The model under review builds one solid part; all positions refer to its coordinate system, in mm. A direction names the side the tool comes from. Coordinates: 2 decimals unless noted, no trailing zeros. Order: outer loops, then holes, each group sorted by start corner. A loop starts at its lowest first (then second) coordinate and runs counter-clockwise, first axis right, second up. Notation, with made-up numbers: (59.25, -20.75) -> (86.25, -20.75) arc R18 ccw to (86.25, -4.75) -> close; hole circle Ø3 at (32, 89). An arc over 180 degrees is marked (long way). Put each result on its own line as item: value.
from build123d import *

# Parameters (mm, degrees)
JOTYY_MIRRORED_START         = -10
JOTYY_MIRRORED_OUTLINE_W     = 53.8
JOTYY_MIRRORED_OUTLINE_H     = 36
JOTYY_MIRRORED_OUTLINE_R     = 2.1
JOTYY_MIRRORED_OUTLINE_R_2   = 11
JOTYY_MIRRORED_DEPTH         = 10
JOTYY_MIRRORED_2_OUTLINE_R   = 11
JOTYY_MIRRORED_2_OUTLINE_R_2 = 4
JOTYY_MIRRORED_2_DEPTH       = 2.5
SKETCH1_R                    = 4
CUT_EXTRUDE1_DEPTH           = 10
CUT_EXTRUDE2_DEPTH           = 58.009529002


# Read off the part's stored shape, not the designer's step: jotyy_Mirrored
with BuildPart() as part:
    # jotyy_Mirrored outline → jotyy_Mirrored (new body)
    with BuildSketch(Plane.XY.offset(JOTYY_MIRRORED_START)):
        with Locations((-26.9, 20)):
            Rectangle(JOTYY_MIRRORED_OUTLINE_W, JOTYY_MIRRORED_OUTLINE_H)
        with Locations((-47.5, 7.5)):
            Circle(JOTYY_MIRRORED_OUTLINE_R, mode=Mode.SUBTRACT)
        with Locations((-22.5, 7.5)):
            Circle(JOTYY_MIRRORED_OUTLINE_R, mode=Mode.SUBTRACT)
        with Locations((-5, 7.5)):
            Circle(JOTYY_MIRRORED_OUTLINE_R, mode=Mode.SUBTRACT)
        with Locations((-35, 20)):
            Circle(JOTYY_MIRRORED_OUTLINE_R_2, mode=Mode.SUBTRACT)
        with Locations((-47.5, 32.5)):
            Circle(JOTYY_MIRRORED_OUTLINE_R, mode=Mode.SUBTRACT)
        with Locations((-22.5, 32.5)):
            Circle(JOTYY_MIRRORED_OUTLINE_R, mode=Mode.SUBTRACT)
        with Locations((-5, 32.5)):
            Circle(JOTYY_MIRRORED_OUTLINE_R, mode=Mode.SUBTRACT)
    extrude(amount=JOTYY_MIRRORED_DEPTH)

    # jotyy_Mirrored 2 outline → jotyy_Mirrored 2 (add)
    with BuildSketch(Plane.XY.offset(JOTYY_MIRRORED_START)):
        with Locations((-35, 20)):
            Circle(JOTYY_MIRRORED_2_OUTLINE_R)
        with Locations((-35, 20)):
            Circle(JOTYY_MIRRORED_2_OUTLINE_R_2, mode=Mode.SUBTRACT)
    extrude(amount=JOTYY_MIRRORED_2_DEPTH)

    # Sketch1 → Cut-Extrude1 (cut)
    with BuildSketch(Plane.XY):
        with Locations((-10, 20)):
            Circle(SKETCH1_R)
    extrude(amount=-CUT_EXTRUDE1_DEPTH, mode=Mode.SUBTRACT)

    # Sketch4 → Cut-Extrude2 (cut, through all)
    with BuildSketch(Plane(origin=(-6.022770261, 7.876766856, -7.746840682), x_dir=(-0.8770067574433524, -0.3073815854436153, 0.36929081809444725), z_dir=(-0.4786451376421942, 0.6259870446034146, -0.6156614753256595))):
        Polygon((61.660399682, 43.281573414), (-67.322963421, -199.854992021), (-184.813959978, -137.526300969), (-55.830596875, 105.610264465), align=None)
    extrude(amount=-CUT_EXTRUDE2_DEPTH, mode=Mode.SUBTRACT)


solid = part.part
Item 1: Consider section B-B on x = -35. Write out the cut boundary in (y, z), and give its area (3 significant figures).
Answers below:
outline: (2, -10) -> (16, -10) -> (16, -7.5) -> (9, -7.5) -> (9, 0) -> (2, 0) -> close; (24, -10) -> (38, -10) -> (38, 0) -> (31, 0) -> (31, -7.5) -> (24, -7.5) -> close
area: 175 mm^2
Item 2: Consider section D-D on y = 18. Write out the cut boundary in (x, z).
Answers below:
outline: (-53.8, -10) -> (-38.46, -10) -> (-38.46, -7.5) -> (-45.82, -7.5) -> (-45.82, 0) -> (-53.8, 0) -> close; (-31.54, -10) -> (-13.46, -10) -> (-13.46, 0) -> (-24.18, 0) -> (-24.18, -7.5) -> (-31.54, -7.5) -> close; (-6.54, -10) -> (0, -10) -> (0, -2.14) -> (-2.75, 0) -> (-6.54, 0) -> close
Item 3: Mouldability with a two-part tool opening along Y and no side actions: class faces 1 (the cylindrical face through (-5.46, 30.45, -5.07)), 2 (the flat face through (0, 27, -5)), 3 (the flat face through (-9.302, 8.195, -4.874)) as +Y half, -Y half, draft (parallel to the pull), parting line (faces both ways), or undercut.
Answers below:
face 1: undercut
face 2: draft
face 3: -Y half
Item 4: For faces 4 (the flat face through (-27, 20, -10)), 5 (the flat face through (-35, 15, -7.5)), list the 3-axis set-ups (+Z, -Z, +X, -X, +Y, -Y) from which the entire face can be reached by the end or side of a thin tool; tool diameter is ignored.
Answers below:
face 4: -Z, +X, -X, +Y, -Y
face 5: +Z
Item 5: Consider section A-A on y = 32.5. Write out the cut boundary in (x, z), and give its area (3 significant figures).
Answers below:
outline: (-53.8, -10) -> (-49.6, -10) -> (-49.6, 0) -> (-53.8, 0) -> close; (-45.4, -10) -> (-24.6, -10) -> (-24.6, 0) -> (-45.4, 0) -> close; (-20.4, -10) -> (-7.1, -10) -> (-7.1, 0) -> (-20.4, 0) -> close; (-2.9, -10) -> (0, -10) -> (0, 0) -> (-2.9, 0) -> close
area: 412 mm^2
Item 6: For pin 1 Ø1 at (y, z) = (7.5, -2.5) entering from +X; pin 2 Ø1 at (x, y) = (-9, 21.5) entering from -Z; pin 3 Ø1 at (y, z) = (7.5, -1.5) entering from +X, all flat-tipped, find the tip position at first contact; note any pin that passes through.
Answers below:
pin 1: x = -12.35
pin 2: through
pin 3: x = -13.63
Item 7: Consider section C-C on x = -47.5. Write out the cut boundary in (y, z).
Answers below:
outline: (2, -10) -> (5.4, -10) -> (5.4, 0) -> (2, 0) -> close; (9.6, -10) -> (30.4, -10) -> (30.4, 0) -> (9.6, 0) -> close; (34.6, -10) -> (38, -10) -> (38, 0) -> (34.6, 0) -> close
Item 8: For line 1 (Y direction, x = -22.5, z = -5.75); line 2 (Y direction, x = -5, z = -9); line 3 (Y direction, x = -35, z = -4.75), list the stretches that pass through material, from the lowest coordinate up. Write a range as from..to.
Answers below:
line 1: 2..5.4, 9.6..30.4, 34.6..38
line 2: 9.6..30.4, 34.6..38
line 3: 2..9, 31..38
